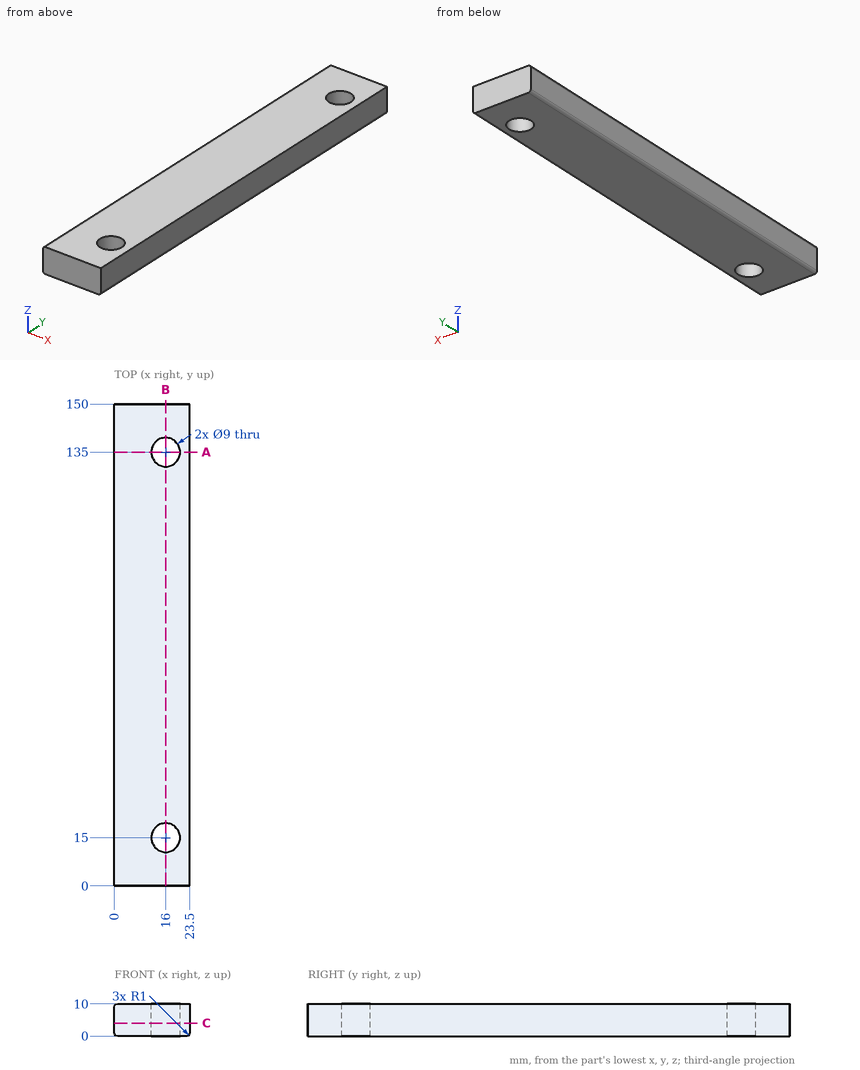
Job drawing, mm, ordinate dimensions from the low corner. One solid piece. Round coordinates to 2 decimals unless told otherwise and drop trailing zeros. Write each loop counter-clockwise with the first axis right and the second up, starting at its lowest first coordinate (ties: lowest second). Pieces come first, ordered by that corner, then holes.
1) Band-saw the part on A-A, the plane y = 135. List the corners of the cut face in (x, z), and give its area (3 significant figures).
2) Band-saw the part on C-C, the plane z = 4. List the corners of the cut face in (x, y).
3) Pin check, flat tips, straight feed: pin 1 (10.5 mm diameter, centred on x = 16, y = 135, fed in from -Z); pin 2 (7 mm diameter, centred on x = 16, y = 15, fed in from -Z). Stop position of each tip, or through.
4) Band-saw the part on B-B, the plane x = 16. List the corners of the cut face in (y, z).
5) Drill centre lines: probe 1 along Y at (x, z) = (16, 3); probe 2 along Y at (x, z) = (14.5, 2.25); probe 3 along X at (y, z) = (16, 1.75). Where is each one in solid material? Low to high.
Ans:
1. outline: (0, 1) arc R1 ccw to (1, 0) - (11.5, 0) - (11.5, 10) - (1, 10) arc R1 ccw to (0, 9) - close; (20.5, 0) - (22.5, 0) arc R1 ccw to (23.5, 1) - (23.5, 10) - (20.5, 10) - close
1. area: 144 mm2
2. outline: (0, 0) - (23.5, 0) - (23.5, 150) - (0, 150) - close; hole circle Ø9 at (16, 15); hole circle Ø9 at (16, 135)
3. pin 1: stops at z = 0
3. pin 2: passes through
4. outline: (0, 0) - (10.5, 0) - (10.5, 10) - (0, 10) - close; (19.5, 0) - (130.5, 0) - (130.5, 10) - (19.5, 10) - close; (139.5, 0) - (150, 0) - (150, 10) - (139.5, 10) - close
5. probe 1: y = 0 to 10.5, 19.5 to 130.5, 139.5 to 150
5. probe 2: y = 0 to 10.76, 19.24 to 130.76, 139.24 to 150
5. probe 3: x = 0 to 11.61, 20.39 to 23.5
